```python
from build123d import *

# Parameters (mm, degrees)
F1_DEPTH = 3
F0_W     = 50
F0_H     = 75
F2_DEPTH = 1.5
F3_DEPTH = 5


with BuildPart() as f1:
    # F0 (on Top) → F1 (new body)
    with BuildSketch(Plane.XY):
        Polygon((55, -5), (55, 0), (55, 85), (-5, 85), (-5, 0), (-5, -5), align=None)
        Polygon((51, 76), (51, 0), (51, -1), (-1, -1), (-1, 76), align=None, mode=Mode.SUBTRACT)
        with BuildLine():
            Line((-5, 85), (55, 85))
            ThreePointArc((55, 85), (25, 115), (-5, 85))
        make_face()
    extrude(amount=F1_DEPTH)



with BuildPart() as f2:
    # F0 (on Top) → F2 (new body)
    with BuildSketch(Plane.XY):
        with Locations((25, 37.5)):
            Rectangle(F0_W, F0_H)
    extrude(amount=F2_DEPTH)


with BuildPart() as f1_1:
    add(f1.part)

    add(f2.part)  # F3 merges F2
    # F0 (on Top) → F3 (join)
    with BuildSketch(Plane.XY):
        Polygon((51, -1), (51, 0), (51, 76), (-1, 76), (-1, -1), align=None)
        with Locations((25, 37.5)):
            Rectangle(F0_W, F0_H, mode=Mode.SUBTRACT)
    extrude(amount=F3_DEPTH)


solid = f1_1.part
```
Verification items for the finished model (mm, model axes). A direction names the side the tool comes from. Coordinates: 2 decimals unless noted, no trailing zeros. Write each loop counter-clockwise with the first axis right and the second up, starting at its lowest first coordinate (ties: lowest second). Pieces come first, ordered by that corner, then holes. Notation, with made-up numbers: M 73.5,62.5 L 122.5,62.5 A28 cw 122.5,88.5 Z; hole C -40,-7 d7. An arc over 180 degrees is marked long. Answer as a JSON object with one key per item and string values. Group by question number.
(1) Tool access check on faces 1 (the face through (25.66, 114.993, 1.479)), 2 (the face through (50, 37, 3)). Record the directions out of +Z, -Z, +X, -X, +Y, -Y that give a thin tool (end or side, any length) a straight path to the whole face; none if there is none.
(2) Material ranges on line 1 (X direction, y = 53, z = 2); line 2 (Y direction, x = 38, z = 4.6); line 3 (X direction, y = 20.5, z = 4.2), recorded low to high.
(3) Cross-section at C-C, the plane x = 25. Record the cut outline in (y, z), and give its area (4 significant figures).
(4) Cross-section at A-A, the plane z = 4.2. Record the cut outline in (x, y).
(5) Cross-section at B-B, the plane y = 57.5. Record the cut outline in (x, z), and give its area (3 significant figures).
(6) Gauge pin test, flat ends, axial feed: pin 1 (1 mm diameter, centred on x = 29, z = 4, fed in from +Y); pin 2 (0.6 mm diameter, centred on x = 18.5, z = 4, fed in from -Y); pin 3 (3 mm diameter, centred on x = 36, y = 42, fed in from +Z). Record the tip position at first contact, or that the pin passes through.
(7) Release check for a two-part mould opening along X. For faces 3 (the face through (55, 39, 1)), 4 (the face through (-0.2, 37.7, 5)), 5 (the face through (25, 0, 3)) record: +X half, -X half, draft (parallel to the pull), parting line (faces both ways), or undercut.
Reply:
{
 "1": {"face 1": "+Z, -Z, +Y", "face 2": "+Z"},
 "2": {"line 1": "-5 to 0, 50 to 55", "line 2": "-1 to 0, 75 to 76", "line 3": "-1 to 0, 50 to 51"},
 "3": {"outline": "M -5,0 L 115,0 L 115,3 L 76,3 L 76,5 L 75,5 L 75,1.5 L 0,1.5 L 0,5 L -1,5 L -1,3 L -5,3 Z", "area": "251.5 mm²"},
 "4": {"outline": "M -1,-1 L 51,-1 L 51,76 L -1,76 Z; hole M 0,0 L 50,0 L 50,75 L 0,75 Z"},
 "5": {"outline": "M -5,0 L 55,0 L 55,3 L 51,3 L 51,5 L 50,5 L 50,1.5 L 0,1.5 L 0,5 L -1,5 L -1,3 L -5,3 Z", "area": "109 mm²"},
 "6": {"pin 1": "y = 76", "pin 2": "y = -1", "pin 3": "z = 1.5"},
 "7": {"face 3": "+X half", "face 4": "draft", "face 5": "undercut"}
}
